Work out the finished part from the listing and answer in its coordinate system (mm). A direction names the side the tool comes from. Round coordinates to 2 decimals unless told otherwise and drop trailing zeros. Loops run counter-clockwise (first coordinate to the right, second up) from the corner with the lowest first, then second, coordinate; pieces in that order, holes last. Notation, with made-up numbers: (29, 33) - (44, 33) arc R20 ccw to (44, 59) - close; hole circle Ø4 at (45, 82). An arc over 180 degrees is marked (long way). Use CSV: the item, a comma, the result in double quotes. Start each with the question number.
from build123d import *

# Parameters (mm, degrees)
SKETCH1_R           = 6.5
SKETCH1_R_2         = 4
BOSS_EXTRUDE1_DEPTH = 12
BOSS_EXTRUDE2_START = -3
SKETCH2_R           = 0.75
BOSS_EXTRUDE2_DEPTH = 3
SKETCH4_R           = 6.5
SKETCH4_R_2         = 5
CUT_EXTRUDE1_DEPTH  = 2
BOSS_EXTRUDE4_START = -10
BOSS_EXTRUDE4_DEPTH = 10
CHAMFER1_SIZE       = 1.5


with BuildPart() as part:
    # Sketch1 → Boss-Extrude1 (new body)
    with BuildSketch(Plane(origin=(0, 0, 0), x_dir=(1, 0, 0), z_dir=(0, 1, 0))):
        with Locations(Location((0, 0, 0), (0, 0, 270))):
            Circle(SKETCH1_R)
        with Locations(Location((0, 0, 0), (0, 0, 270))):
            Circle(SKETCH1_R_2, mode=Mode.SUBTRACT)
    extrude(amount=BOSS_EXTRUDE1_DEPTH)

    # Sketch2 → Boss-Extrude2 (add)
    with BuildSketch(Plane(origin=(0, 12, 0), x_dir=(1, 0, 0), z_dir=(0, 1, 0)).offset(BOSS_EXTRUDE2_START)):
        with BuildLine():
            Line((22.477272727, 2.961791813), (1.034090909, 6.417215595))
            ThreePointArc((1.034090909, 6.417215595), (4.948312384, 4.214760319), (6.5, 0))
            ThreePointArc((6.5, 0), (4.948312384, -4.214760319), (1.034090909, -6.417215595))
            Line((1.034090909, -6.417215595), (22.477272727, -2.961791813))
            ThreePointArc((22.477272727, -2.961791813), (25, 0), (22.477272727, 2.961791813))
        make_face()
        with Locations(Location((22, 0, 0), (0, 0, 270))):
            Circle(SKETCH2_R, mode=Mode.SUBTRACT)
    extrude(amount=BOSS_EXTRUDE2_DEPTH)

    # Sketch4 → Cut-Extrude1 (cut)
    with BuildSketch(Plane.XZ):
        with Locations(Location((0, 0, 0), (0, 0, 270))):
            Circle(SKETCH4_R)
        with Locations(Location((0, 0, 0), (0, 0, 270))):
            Circle(SKETCH4_R_2, mode=Mode.SUBTRACT)
    extrude(amount=-CUT_EXTRUDE1_DEPTH, mode=Mode.SUBTRACT)

    # Sketch5 → Boss-Extrude4 (add)
    with BuildSketch(Plane(origin=(0, 12, 0), x_dir=(1, 0, 0), z_dir=(0, 1, 0)).offset(BOSS_EXTRUDE4_START)):
        with BuildLine():
            Line((-3.726313009, -1.454163457), (-0.60381401, 3.954163457))
            ThreePointArc((-0.60381401, 3.954163457), (-3.464101615, 2), (-3.726313009, -1.454163457))
        make_face()
    extrude(amount=BOSS_EXTRUDE4_DEPTH)

    # Chamfer1
    chamfer1_edges = [part.edges().sort_by_distance(p)[0] for p in [
        (0, 2, 5),
    ]]
    chamfer(chamfer1_edges, length=CHAMFER1_SIZE - 0.0001)  # a hair under: the kernel refuses the full size


solid = part.part
Item 1: The mould has two halves that part along Z. Classify faces 3 (the cylindrical face through (-4.88, 0.25, 1.08)), 4 (the flat face through (-2.19, 6.93, -1.21)), 5 (the flat face through (13, 9, 0)): pulls with the +Z half, pulls with the -Z half, needs draft (parallel to the pull), parting line crosses it, or undercut.
Item 2: A cutting plane is placed at B-B (z = 0). State how many separate pieces and enclosed holes the cut face has, plus the area to 3 significant figures.
Item 3: Find the intervals of material crossed by probe 1 along X at (y, z) = (10.6, 0); probe 2 along Z at (x, y) = (0, 3); probe 3 along Z at (x, y) = (3.5, 4.25), in increasing order. Write a range as [from, to].
Item 4: A cutting plane is placed at D-D (x = 22). Determine the outline of the cut face in (y, z).
Item 5: A cutting plane is placed at C-C (y = 3.5). Determine the outline of the cut face in (x, z), plus the area to 3 significant figures.
Item 6: Each of these flat-tipped pins is pushed along its axis until it touches: pin 1 Ø2 at (y, z) = (10.5, -4) entering from -X; pin 2 Ø1 at (x, z) = (9, 2.5) entering from -Y; pin 3 Ø6 at (x, y) = (7, 3.5) entering from -Z. Where does it stop, or does it pass through?
Item 7: Which of the six approach directions +Z, -Z, +X, -X, +Y, -Y give full straight-line access (tool end or side, diameter ignored) to faces 1 (the flat face through (9, 12, 0)), 2 (the flat face through (-3, 2, -1))?
Result sheet:
1,face 3,"parting line crosses it"
1,face 4,"undercut"
1,face 5,"needs draft"
2,separate pieces,"3"
2,enclosed holes,"0"
2,area,"118 mm^2"
3,probe 1,"[-6.5, -2.89], [4, 21.25], [22.75, 25]"
3,probe 2,"[-6.5, -4], [4, 6.5]"
3,probe 3,"[-5.48, -1.94], [1.94, 5.48]"
4,outline,"(9, -3.04) - (12, -3.04) - (12, -0.75) - (9, -0.75) - close; (9, 0.75) - (12, 0.75) - (12, 3.04) - (9, 3.04) - close"
5,outline,"circle Ø13 at (0, 0); hole (-3.73, 1.45) - (-0.6, -3.95) arc R4 ccw (long way) to start"
5,area,"89.0 mm^2"
6,pin 1,"x = -5.77"
6,pin 2,"y = 9"
6,pin 3,"z = -5.12"
7,face 1,"+Z, -Z, +X, -X, +Y"
7,face 2,"-Y"
